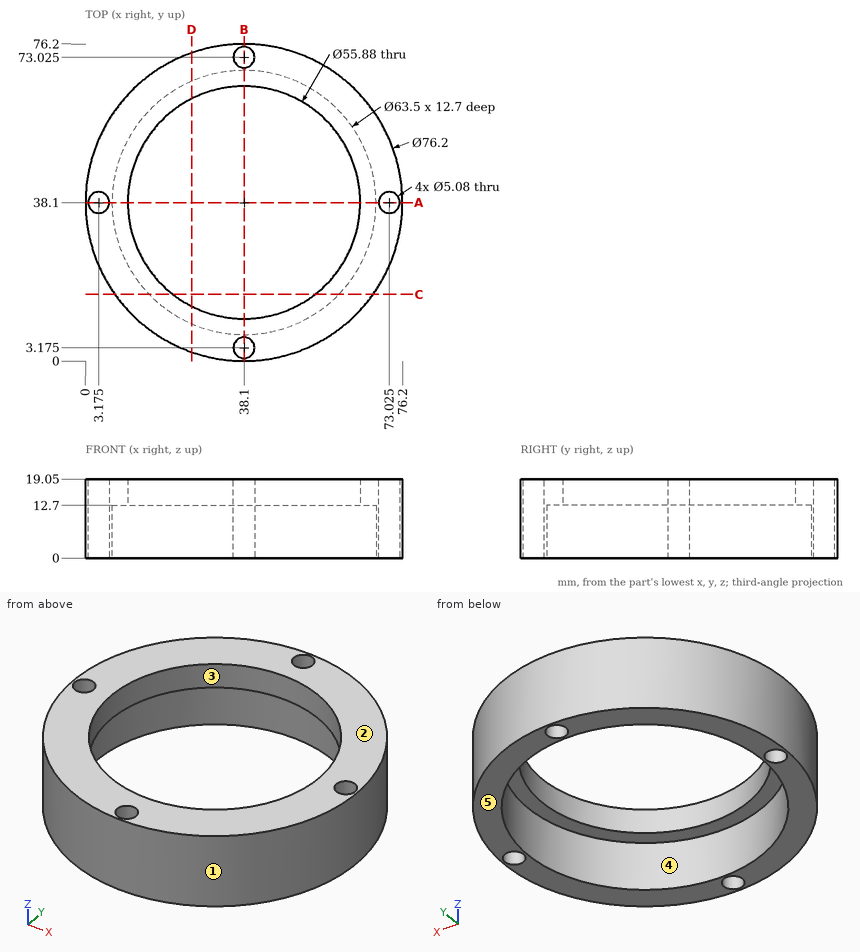
Job drawing, mm, ordinate dimensions from the low corner. One solid piece. A direction names the side the tool comes from. Round coordinates to 2 decimals unless told otherwise and drop trailing zeros. Loops run counter-clockwise (first coordinate to the right, second up) from the corner with the lowest first, then second, coordinate; pieces in that order, holes last. Notation, with made-up numbers: (6.5, -34.5) -> (23.5, -34.5) arc R14 ccw to (23.5, -21.5) -> close; hole circle Ø10 at (-29, 33). An arc over 180 degrees is marked (long way). One line per item, written item: value. Start each with the question number.
Q1. Cut at A-A on y = 38.1. List the corners of the cut face in (x, z) (3 decimals), plus the area to 3 significant figures.
Q2. 3-axis set-ups, long thin cutter, end or side, ignore diameter. For the marked faces 4 and 5: which of +Z, -Z, +X, -X, +Y, -Y reach the whole face in a straight line?
Q3. Cut at D-D on x = 25.5. List the corners of the cut face in (y, z), plus the area to 3 significant figures.
Q4. Two-plate mould, pull along Y, no slides. Class the marked faces 1, 2 and 3: released by +Y, released by -Y, zero draft, split by the parting line, or undercut.
Q5. Probe line 1 along Y through (x, z) = (38.1, 13.75) (3 decimals); line 2 along X through (y, z) = (38, 15); line 3 along Y through (x, z) = (38.1, 9) (3 decimals). List the from-to ranges inside material, lowest first.
Q6. Cut at C-C on y = 16. List the corners of the cut face in (x, z), plus the area to 3 significant figures.
Q7. Drop flat-ended pins along their axis: pin 1 Ø8 at (y, z) = (24, 14) entering from -X; pin 2 Ø3 at (x, z) = (67, 12) entering from +Y; pin 3 Ø3 at (y, z) = (36.5, 15) entering from +X. Give the stop position or say it passes through.
Computed:
1. outline: (0, 0) -> (0.635, 0) -> (0.635, 19.05) -> (0, 19.05) -> close; (5.715, 0) -> (6.35, 0) -> (6.35, 12.7) -> (10.16, 12.7) -> (10.16, 19.05) -> (5.715, 19.05) -> close; (66.04, 12.7) -> (69.85, 12.7) -> (69.85, 0) -> (70.485, 0) -> (70.485, 19.05) -> (66.04, 19.05) -> close; (75.565, 0) -> (76.2, 0) -> (76.2, 19.05) -> (75.565, 19.05) -> close
1. area: 96.8 mm²
2. face 4: -Z
2. face 5: -Z, +X, -X, +Y, -Y
3. outline: (2.14, 0) -> (8.96, 0) -> (8.96, 12.7) -> (13.16, 12.7) -> (13.16, 19.05) -> (2.14, 19.05) -> close; (63.04, 12.7) -> (67.24, 12.7) -> (67.24, 0) -> (74.06, 0) -> (74.06, 19.05) -> (63.04, 19.05) -> close
3. area: 313 mm²
4. face 1: split by the parting line
4. face 2: zero draft
4. face 3: undercut
5. line 1: 0 to 0.635, 5.715 to 10.16, 66.04 to 70.485, 75.565 to 76.2
5. line 2: 0 to 0.64, 5.71 to 10.16, 66.04 to 70.49, 75.56 to 76.2
5. line 3: 0 to 0.635, 5.715 to 6.35, 69.85 to 70.485, 75.565 to 76.2
6. outline: (7.06, 0) -> (15.3, 0) -> (15.3, 12.7) -> (21.01, 12.7) -> (21.01, 19.05) -> (7.06, 19.05) -> close; (55.19, 12.7) -> (60.9, 12.7) -> (60.9, 0) -> (69.14, 0) -> (69.14, 19.05) -> (55.19, 19.05) -> close
6. area: 386 mm²
7. pin 1: x = 1.36
7. pin 2: y = 64.57
7. pin 3: x = 76.2
